```python
from build123d import *

# Parameters (mm, degrees)
EXTRUDE_1_DEPTH     = 10
SKETCH_2_W          = 10
SKETCH_2_H          = 7.5
SKETCH_2_W_2        = 1.5
CUT_EXTRUDE_1_DEPTH = 10
CUT_EXTRUDE_START   = -1.5
SKETCH_3_W          = 13
SKETCH_3_H          = 7.5
CUT_EXTRUDE_2_DEPTH = 20
CUT_EXTRUDE_3_REACH = 17.564
SKETCH_4_W          = 5.5
SKETCH_4_H          = 20
FILLET_1_R          = 2.5
FILLET_2_R          = 1
SKETCH_5_R          = 1.6
CUT_EXTRUDE_4_DEPTH = 20
MOVE_START          = -6.5
MOVE_FACE_1_DEPTH   = 13
MOVE_FACE_2_BY      = 0.3
MOVE_FACE_2_2_BY    = 0.3


# Read off the part's stored shape, not the designer's step: 面の移動1
with BuildPart() as part:
    # ｽｹｯﾁ1 → ﾎﾞｽ - 押し出し1 (new, symmetric)
    with BuildSketch(Plane.XY):
        with BuildLine():
            Line((-5, 5), (5, 5))
            Line((5, 5), (5, -5))
            Line((5, -5), (6.5, -5))
            Line((6.5, -5), (6.5, 6.5))
            Line((6.5, 6.5), (4.062019202, 6.5))
            ThreePointArc((4.062019202, 6.5), (0, 12), (-4.062019202, 6.5))
            Line((-4.062019202, 6.5), (-6.5, 6.5))
            Line((-6.5, 6.5), (-6.5, -5))
            Line((-6.5, -5), (-5, -5))
            Line((-5, -5), (-5, 5))
        make_face()
        with BuildLine():
            Line((2.449489743, 6.5), (-2.449489743, 6.5))
            ThreePointArc((-2.449489743, 6.5), (0, 10.5), (2.449489743, 6.5))
        make_face(mode=Mode.SUBTRACT)
    extrude(amount=EXTRUDE_1_DEPTH, both=True)

    # ｽｹｯﾁ2 → ｶｯﾄ - 押し出し1 (cut)
    with BuildSketch(Plane.XZ.offset(5)):
        Rectangle(SKETCH_2_W, SKETCH_2_H)
        with Locations((-5.75, 0)):
            Rectangle(SKETCH_2_W_2, SKETCH_2_H)
        with Locations((5.75, 0)):
            Rectangle(SKETCH_2_W_2, SKETCH_2_H)
    extrude(amount=-CUT_EXTRUDE_1_DEPTH, mode=Mode.SUBTRACT)

    # ｽｹｯﾁ3 → ｶｯﾄ - 押し出し2 (cut)
    with BuildSketch(Plane.XZ.offset(-5).offset(CUT_EXTRUDE_START)):
        Rectangle(SKETCH_3_W, SKETCH_3_H)
    extrude(amount=-CUT_EXTRUDE_2_DEPTH, mode=Mode.SUBTRACT)

    # ｽｹｯﾁ4 → ｶｯﾄ - 押し出し3 (cut, up to next)
    with BuildSketch(Plane.XZ.offset(-5), mode=Mode.PRIVATE) as cut_extrude_3_sk1:
        Rectangle(SKETCH_4_W, SKETCH_4_H)
    cut_extrude_3_tool1 = extrude(cut_extrude_3_sk1.sketch, amount=-CUT_EXTRUDE_3_REACH, mode=Mode.PRIVATE) & part.part
    add(cut_extrude_3_tool1.solids().sort_by_distance((0, 5, 0))[0], mode=Mode.SUBTRACT)

    # ﾌｨﾚｯﾄ1
    fillet_1_edges = [part.edges().sort_by_distance(p)[0] for p in [
        (5.75, -5, -10),
        (-5.75, -5, -10),
        (-5.75, -5, 10),
        (-5.75, -5, -3.75),
        (-5.75, -5, 3.75),
        (5.75, -5, -3.75),
        (5.75, -5, 3.75),
        (5.75, -5, 10),
    ]]
    fillet(fillet_1_edges, radius=FILLET_1_R)

    # ﾌｨﾚｯﾄ2
    fillet_2_edges = [part.edges().sort_by_distance(p)[0] for p in [
        (-4.062019202, 6.5, 6.875),
        (4.062019202, 6.5, 6.875),
        (-4.062019202, 6.5, -6.875),
        (4.062019202, 6.5, -6.875),
    ]]
    fillet(fillet_2_edges, radius=FILLET_2_R)

    # ｽｹｯﾁ5 → ｶｯﾄ - 押し出し4 (cut)
    with BuildSketch(Plane.ZY.offset(6.5)):
        with Locations((-6.875, 0)):
            Circle(SKETCH_5_R)
    cut_extrude_4 = extrude(amount=-CUT_EXTRUDE_4_DEPTH, mode=Mode.SUBTRACT)

    # ﾐﾗｰ1: ｶｯﾄ - 押し出し4 across plane
    add(cut_extrude_4.mirror(Plane.XY), mode=Mode.SUBTRACT)

    # Move Face 1 outline → Move Face 1 (cut)
    with BuildSketch(Plane.YZ.offset(MOVE_START)):
        with BuildLine():
            ThreePointArc((-1, 3.75), (-2.767766953, 4.482233047), (-3.5, 6.25))
            Line((-3.5, 6.25), (-3.5, 7.5))
            ThreePointArc((-3.5, 7.5), (-2.767766953, 9.267766953), (-1, 10))
            Line((-1, 10), (-2.5, 10))
            ThreePointArc((-2.5, 10), (-4.267766953, 9.267766953), (-5, 7.5))
            Line((-5, 7.5), (-5, 6.25))
            ThreePointArc((-5, 6.25), (-4.267766953, 4.482233047), (-2.5, 3.75))
            Line((-2.5, 3.75), (-1, 3.75))
        make_face()
        with BuildLine():
            ThreePointArc((-1, -10), (-2.767766953, -9.267766953), (-3.5, -7.5))
            Line((-3.5, -7.5), (-3.5, -6.25))
            ThreePointArc((-3.5, -6.25), (-2.767766953, -4.482233047), (-1, -3.75))
            Line((-1, -3.75), (-2.5, -3.75))
            ThreePointArc((-2.5, -3.75), (-4.267766953, -4.482233047), (-5, -6.25))
            Line((-5, -6.25), (-5, -7.5))
            ThreePointArc((-5, -7.5), (-4.267766953, -9.267766953), (-2.5, -10))
            Line((-2.5, -10), (-1, -10))
        make_face()
    extrude(amount=MOVE_FACE_1_DEPTH, mode=Mode.SUBTRACT)

    # Move Face 2: a curved face moved outward by 0.3
    add(Solid.thicken(part.faces().sort_by_distance((-5.75, 0, -8.475))[0], MOVE_FACE_2_BY))

    # Move Face 2 2: a curved face moved outward by 0.3
    add(Solid.thicken(part.faces().sort_by_distance((-5.75, 0, 8.475))[0], MOVE_FACE_2_2_BY))


solid = part.part
```
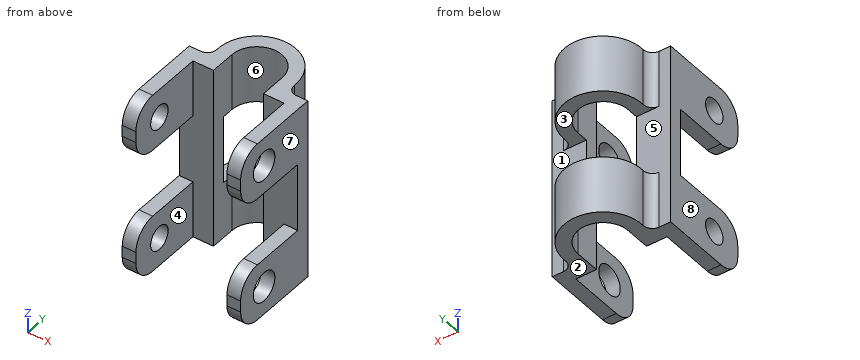
Could you check a few things on this model? Use its own coordinates, in mm. Face numbers are marked on the shaded views. A direction names the side the tool comes from. Round coordinates to 2 decimals unless told otherwise and drop trailing zeros. Loops run counter-clockwise (first coordinate to the right, second up) from the corner with the lowest first, then second, coordinate; pieces in that order, holes last. Notation, with made-up numbers: (13, -29.75) -> (47, -29.75) arc R33 ccw to (47, 9.25) -> close; hole circle Ø8 at (-11, -10.75). An arc over 180 degrees is marked (long way). Put each result on its own line as item: value.
Q1. For pin 1 Ø4 at (y, z) = (0, 6.875) entering from -X; pin 2 Ø1.5 at (x, z) = (-4, 8) entering from -Y; pin 3 Ø2 at (x, z) = (2, 3) entering from +Y, each with a flat end and sliding along its axis, tell me the tip position at first contact or that it passes through.
Checks:
pin 1: x = -6.5
pin 2: y = 5
pin 3: y = 11.78
Q2. I want a section at D-D on y = 4.75. Write out the boundary of the cut face in (x, z).
Checks:
outline: (-6.5, -10) -> (-5, -10) -> (-5, -3.75) -> (-6.5, -3.75) -> close; (-6.5, 3.75) -> (-5, 3.75) -> (-5, 10) -> (-6.5, 10) -> close; (5, -10) -> (6.5, -10) -> (6.5, -3.75) -> (5, -3.75) -> close; (5, 3.75) -> (6.5, 3.75) -> (6.5, 10) -> (5, 10) -> close
Q3. Which directions (+Z, -Z, +X, -X, +Y, -Y) give clear straight access to the entire face, cutting with the end or side of a thin tool? Please do the marked faces 1, 2, 3, 4 and 5.
Checks:
face 1: +X, +Y
face 2: -Z, +X, -X, +Y, -Y
face 3: +X, -X, +Y
face 4: +Z, -Z, -Y
face 5: -X, +Y
Q4. Please list where these lines run through material, in increasing order: line 1 (Z direction, x = -2, y = 10); line 2 (X direction, y = 3.25, z = 5.5); line 3 (X direction, y = 5.75, z = -6). Write a range as from..to.
Checks:
line 1: -10..-3.75, 3.75..10
line 2: -6.5..-5, 5..6.5
line 3: -6.5..-2.75, 2.75..6.5
Q5. I want a section at B-B on y = 0. Give the number of separate pieces and of enclosed holes in the cut face, and give its area (3 significant figures).
Checks:
separate pieces: 8
enclosed holes: 0
area: 20.1 mm2
Q6. I want a section at C-C on z = -2.5. Write out the boundary of the cut face in (x, y), and give its area (4 significant figures).
Checks:
outline: (-6.5, 5) -> (-2.75, 5) -> (-2.75, 6.5) -> (-6.5, 6.5) -> close; (2.75, 5) -> (6.5, 5) -> (6.5, 6.5) -> (2.75, 6.5) -> close
area: 11.25 mm2
Q7. Thinking about a two-plate mould opening in X: for the marked faces 6, 7 and 8, which applies, pulls with the +X half, pulls with the -X half, needs draft (parallel to the pull), parting line crosses it, or undercut?
Checks:
face 6: undercut
face 7: pulls with the +X half
face 8: pulls with the -X half
Q8. I want a section at A-A on x = 0. Write out the boundary of the cut face in (y, z), and give its area (4 significant figures).
Checks:
outline: (10.5, -10) -> (12, -10) -> (12, -3.75) -> (10.5, -3.75) -> close; (10.5, 3.75) -> (12, 3.75) -> (12, 10) -> (10.5, 10) -> close
area: 18.75 mm2
